Part print with two shaded views. Sizes in mm from the minimum x, y, z corner. A direction names the side the tool comes from. Round coordinates to 2 decimals unless told otherwise and drop trailing zeros. Order: outer loops, then holes, each group sorted by start corner. A loop starts at its lowest first (then second) coordinate and runs counter-clockwise, first axis right, second up. Notation, with made-up numbers: (-26, 65) -> (27, 65) arc R25 ccw to (27, 94) -> close; hole circle Ø3 at (79, -22.5). An arc over 180 degrees is marked (long way). Put each result on its own line as item: value. Start each with the question number.
Q1. Pull direction Y, two halves, no side cores. Call the marked faces 4, 5 and 6: released by +Y, released by -Y, zero draft, split by the parting line, or undercut.
Q2. Cut at C-C, the plane x = 3.5. List the corners of the cut face in (y, z).
Q3. Probe L1, parallel to Y at x = 5.5, z = 3; L2, parallel to X at y = 3.5, z = 5; L3, parallel to X at y = 8, z = 2.75. List the from-to ranges inside material, lowest first.
Q4. Cut at B-B, the plane y = 5. List the corners of the cut face in (x, z).
Q5. Flat gauge pins, fed straight in: P1, Ø1.5, axis at x = 1.5, y = 5, coming from the -Z side; P2, Ø4, axis at x = 7, y = 5.5, coming from the +Z side; P3, Ø6, axis at x = 7, z = 2.5, coming from the +Y side; P4, Ø2.5, axis at y = 5, z = 4.5, coming from the -X side. Where does each tip first touch, or does it go through?
Q6. Cut at A-A, the plane x = 0.75. List the corners of the cut face in (y, z), and give its area (3 significant figures).
Q7. 3-axis set-ups, long thin cutter, end or side, ignore diameter. For the marked faces 1, 2 and 3: which of +Z, -Z, +X, -X, +Y, -Y reach the whole face in a straight line?
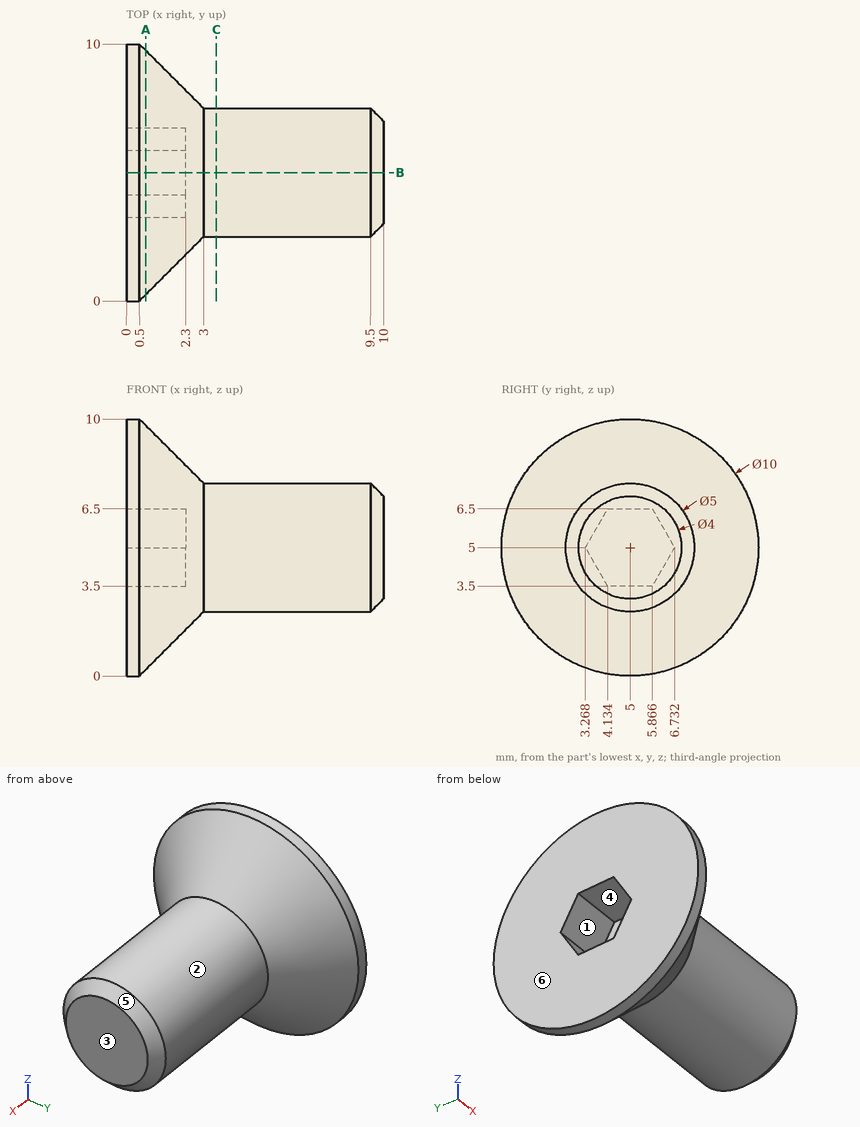
Ans:
1. face 4: undercut
1. face 5: split by the parting line
1. face 6: zero draft
2. outline: circle Ø5 at (5, 5)
3. L1: y = 3.5 to 6.5
3. L2: x = 2.3 to 10
3. L3: x = 0 to 1.75
4. outline: (0, 0) -> (0.5, 0) -> (3, 2.5) -> (9.5, 2.5) -> (10, 3) -> (10, 7) -> (9.5, 7.5) -> (3, 7.5) -> (0.5, 10) -> (0, 10) -> (0, 6.5) -> (2.3, 6.5) -> (2.3, 3.5) -> (0, 3.5) -> close
5. P1: stops at z = 0.25
5. P2: stops at z = 7.5
5. P3: stops at y = 7.5
5. P4: stops at x = 0
6. outline: circle Ø9.5 at (5, 5); hole (3.27, 5) -> (4.13, 3.5) -> (5.87, 3.5) -> (6.73, 5) -> (5.87, 6.5) -> (4.13, 6.5) -> close
6. area: 63.1 mm^2
7. face 1: -X
7. face 2: +X
7. face 3: +Z, -Z, +X, +Y, -Y
